```python
from build123d import *

# Parameters (mm, degrees)
SKETCH1_R           = 2.45
BOSS_EXTRUDE1_DEPTH = 5
BOSS_EXTRUDE2_START = 5
SKETCH2_R           = 4.9
BOSS_EXTRUDE2_DEPTH = 5
FILLET1_R           = 1


with BuildPart() as part:
    # Sketch1 → Boss-Extrude1 (new body)
    with BuildSketch(Plane.XY):
        with BuildLine():
            Line((0, 4.9), (27.899102923, 4.9))
            ThreePointArc((27.899102923, 4.9), (32.799102923, 0), (27.899102923, -4.9))
            Line((27.899102923, -4.9), (0, -4.9))
            ThreePointArc((0, -4.9), (-4.9, 0), (0, 4.9))
        make_face()
        Circle(SKETCH1_R, mode=Mode.SUBTRACT)
    extrude(amount=BOSS_EXTRUDE1_DEPTH)

    # Sketch2 → Boss-Extrude2 (add)
    with BuildSketch(Plane.XY.offset(BOSS_EXTRUDE2_START)):
        with Locations(Location((27.899102923, 0, 0), (0, 0, 90))):
            Circle(SKETCH2_R)
    extrude(amount=BOSS_EXTRUDE2_DEPTH)

    # Fillet1
    # the kernel refuses this fillet: 1 mm, written as the material it takes off along each edge
    with BuildSketch(Plane(origin=(0, 4.9, 5), x_dir=(0, -1, 0), z_dir=(1, 0, 0))) as fillet1_piece_1_section:
        with BuildLine():
            CenterArc((FILLET1_R, FILLET1_R), FILLET1_R, 180, 90)
            Line((0, FILLET1_R), (0, 0))
            Line((0, 0), (FILLET1_R, 0))
        make_face()
    fillet1_piece_1 = extrude(amount=30.399102923, mode=Mode.PRIVATE)
    fillet1_piece_1 = fillet1_piece_1 - Plane(origin=(27.899102923, 0, 4.766386188), x_dir=(0, 1, 0), z_dir=(0, 0, -1)) * Cylinder(4.9, 65, mode=Mode.PRIVATE)
    add(fillet1_piece_1, mode=Mode.SUBTRACT)
    with BuildSketch(Plane(origin=(27.899102923, 0, 10), x_dir=(0, 1, 0), z_dir=(1, 0, 0))) as fillet1_piece_2:
        with BuildLine():
            CenterArc((4.9 - FILLET1_R, -FILLET1_R), FILLET1_R, 0, 90)
            Line((4.9 - FILLET1_R, 0), (4.9, 0))
            Line((4.9, 0), (4.9, -FILLET1_R))
        make_face()
    revolve(axis=Axis((27.899102923, 0, 10), (0, 0, 1)), mode=Mode.SUBTRACT)
    with BuildSketch(Plane(origin=(0, 0, 5), x_dir=(0, -1, 0), z_dir=(1, 0, 0))) as fillet1_piece_3:
        with BuildLine():
            CenterArc((4.9 - FILLET1_R, FILLET1_R), FILLET1_R, 270, 90)
            Line((4.9 - FILLET1_R, 0), (4.9, 0))
            Line((4.9, 0), (4.9, FILLET1_R))
        make_face()
    revolve(axis=Axis((0, 0, 5), (0, 0, -1)), revolution_arc=180, mode=Mode.SUBTRACT)
    with BuildSketch(Plane(origin=(30.399102923, -4.9, 5), x_dir=(0, 0, -1), z_dir=(-1, 0, 0))) as fillet1_piece_4_section:
        with BuildLine():
            CenterArc((FILLET1_R, -FILLET1_R), FILLET1_R, 90, 90)
            Line((0, -FILLET1_R), (0, 0))
            Line((0, 0), (FILLET1_R, 0))
        make_face()
    fillet1_piece_4 = extrude(amount=30.399102923, mode=Mode.PRIVATE)
    fillet1_piece_4 = fillet1_piece_4 - Plane(origin=(27.899102923, 0, 4.766386187), x_dir=(0, 1, 0), z_dir=(0, 0, -1)) * Cylinder(4.9, 65, mode=Mode.PRIVATE)
    add(fillet1_piece_4, mode=Mode.SUBTRACT)


solid = part.part
```
Design review of the part built by this model. Coordinates are the model's own, in mm. A direction names the side the tool comes from. Round coordinates to 2 decimals unless told otherwise and drop trailing zeros. Write each loop counter-clockwise with the first axis right and the second up, starting at its lowest first coordinate (ties: lowest second). Pieces come first, ordered by that corner, then holes.
Item 1: Clearance check with flat-ended pins moving along their axes: pin 1 Ø1.5 at (y, z) = (-3.5, 7.5) entering from -X; pin 2 Ø1 at (y, z) = (-2.5, 3) entering from -X; pin 3 Ø3 at (y, z) = (-2.5, 8) entering from -X. State where each tip first meets the part, or that it passes through.
Item 2: The part is to be moulded in two halves that separate along Y. For faces 1 (the cylindrical face through (-4.9, -0.1, 2)), 2 (the flat face through (11, 0, 5)), 3 (the cylindrical face through (-0.5, -2.4, 2.5)), 4 (the cylindrical face through (13.754, 4.615, 4.699)), say which applies: +Y half, -Y half, draft (parallel to the pull), parting line (faces both ways), or undercut.
Item 3: For faces 5 (the cylindrical face through (32.683, -1.062, 5.437)), 6 (the cylindrical face through (14.145, -4.615, 4.699)), 7 (the flat face through (14, -4.9, 2)), list the 3-axis set-ups (+Z, -Z, +X, -X, +Y, -Y) from which the entire face can be reached by the end or side of a thin tool; tool diameter is ignored.
Item 4: We need section A-A on y = 0. Write out the cut boundary in (x, z).
Item 5: For probe 1 along Y at (x, z) = (0, 2.65); probe 2 along Z at (x, y) = (13, -2.75); probe 3 along X at (y, z) = (0.25, 4.75), list the stretches that pass through material, from the lowest coordinate up.
Item 6: We need section C-C on x = 22. Write out the cut boundary in (y, z), and give its area (3 significant figures).
Item 7: We need section B-B on z = 1.5. Write out the cut boundary in (x, y), and give its area (3 significant figures).
Item 8: We need section D-D on z = 5.75. Write out the cut boundary in (x, y).
Returned:
1. pin 1: stops at x = 23.84
1. pin 2: stops at x = -4.47
1. pin 3: stops at x = 23.1
2. face 1: parting line
2. face 2: draft
2. face 3: undercut
2. face 4: +Y half
3. face 5: +Z
3. face 6: +Z, -X, -Y
3. face 7: +Z, -Z, +X, -X, -Y
4. outline: (-4.9, 0) - (-2.45, 0) - (-2.45, 5) - (-3.9, 5) arc R1 ccw to (-4.9, 4) - close; (2.45, 0) - (32.8, 0) - (32.8, 9) arc R1 ccw to (31.8, 10) - (24, 10) arc R1 ccw to (23, 9) - (23, 5) - (2.45, 5) - close
5. probe 1: y = -4.9 to -2.45, 2.45 to 4.9
5. probe 2: z = 0 to 5
5. probe 3: x = -4.55 to -2.44, 2.44 to 32.79
6. outline: (-4.9, 0) - (4.9, 0) - (4.9, 4) arc R1 ccw to (3.9, 5) - (-3.9, 5) arc R1 ccw to (-4.9, 4) - close
6. area: 48.6 mm2
7. outline: (0, -4.9) - (27.9, -4.9) arc R4.9 ccw to (27.9, 4.9) - (0, 4.9) arc R4.9 ccw to start; hole circle Ø4.9 at (0, 0)
7. area: 330 mm2
8. outline: circle Ø9.8 at (27.9, 0)
